from build123d import *

# Parameters (mm, degrees)
SKETCH1_W           = 25.4
SKETCH1_H           = 82.55
BOSS_EXTRUDE1_DEPTH = 3.175
SKETCH2_W           = 25.4
SKETCH2_H           = 3.175
SKETCH2_H_2         = 60.325
BOSS_EXTRUDE2_DEPTH = 3.175
SKETCH5_W           = 9.525
SKETCH5_H           = 19.05
CUT_EXTRUDE2_DEPTH  = 64.5
SKETCH6_R           = 3.175
CUT_EXTRUDE3_DEPTH  = 89.9


with BuildPart() as part:
    # Sketch1 → Boss-Extrude1 (new body)
    with BuildSketch(Plane.XY):
        Rectangle(SKETCH1_W, SKETCH1_H)
    extrude(amount=BOSS_EXTRUDE1_DEPTH)

    # Sketch2 → Boss-Extrude2 (add)
    with BuildSketch(Plane(origin=(0, 41.275, 0), x_dir=(1, 0, 0), z_dir=(0, 1, 0))):
        with Locations((0, -1.5875)):
            Rectangle(SKETCH2_W, SKETCH2_H)
        with Locations((0, 30.1625)):
            Rectangle(SKETCH2_W, SKETCH2_H_2)
    boss_extrude2 = extrude(amount=BOSS_EXTRUDE2_DEPTH)

    # Sketch5 → Cut-Extrude2 (cut, through all)
    with BuildSketch(Plane.XY.offset(3.175)):
        with Locations((0, 3.175)):
            Rectangle(SKETCH5_W, SKETCH5_H)
    extrude(amount=-CUT_EXTRUDE2_DEPTH, mode=Mode.SUBTRACT)

    # Mirror1: Boss-Extrude2 across plane
    add(boss_extrude2.mirror(Plane.ZX))

    # Sketch6 → Cut-Extrude3 (cut, through all)
    with BuildSketch(Plane(origin=(0, 44.45, 0), x_dir=(1, 0, 0), z_dir=(0, 1, 0))):
        with Locations((0, 49.2125)):
            Circle(SKETCH6_R)
    extrude(amount=-CUT_EXTRUDE3_DEPTH, mode=Mode.SUBTRACT)


solid = part.part
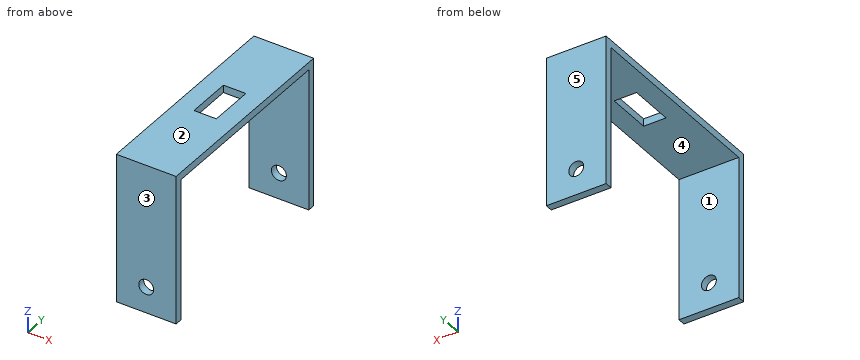
Read the model definition and answer for the solid it produces. Units are mm, in the model's axes. Face numbers are marked on the shaded views. A direction names the side the tool comes from. Round coordinates to 2 decimals unless told otherwise and drop trailing zeros. Write each loop counter-clockwise with the first axis right and the second up, starting at its lowest first coordinate (ties: lowest second). Pieces come first, ordered by that corner, then holes.
1. The part is cut by section D-D, the plane x = -7.75. Determine the outline of the cut face in (y, z) (3 decimals), then the cut area to 3 significant figures.
2. Determine the mould class of the marked faces 3, 4 and 5 for opening direction Y: pulls with the +Y half, pulls with the -Y half, needs draft (parallel to the pull), parting line crosses it, or undercut.
3. The part is cut by section A-A, the plane z = -31.5. Determine the outline of the cut face in (x, y) (3 decimals), then the cut area to 3 significant figures.
4. The part is cut by section B-B, the plane x = 0. State how many separate pieces and enclosed holes the cut face has, then the cut area to 3 significant figures.
5. The part is cut by section C-C, the plane y = -4. Determine the outline of the cut face in (x, z) (1 decimal), then the cut area to 3 significant figures.
6. Straight lines are drawn through the part: L1, parallel to Y at x = 3.25, z = -24 (3 decimals); L2, parallel to Z at x = 0, y = 42.9 (1 decimal); L3, parallel to Z at x = -8, y = -10 (3 decimals). For each, find the intervals that lie inside material, in ascending order.
7. Given pin 1 Ø3 at (x, y) = (-8, 7) entering from -Z; pin 2 Ø8 at (y, z) = (-8, -7) entering from -X, each flat-ended and moving along its own axis, determine where each tip first touches the part or whether it passes through.
8. Which of the six approach directions +Z, -Z, +X, -X, +Y, -Y give full straight-line access (tool end or side, diameter ignored) to the marked faces 1 and 2?
Values:
1. outline: (-44.45, -60.325) - (-41.275, -60.325) - (-41.275, 0) - (41.275, 0) - (41.275, -60.325) - (44.45, -60.325) - (44.45, 3.175) - (-44.45, 3.175) - close
1. area: 665 mm2
2. face 3: pulls with the -Y half
2. face 4: undercut
2. face 5: pulls with the +Y half
3. outline: (-12.7, -44.45) - (12.7, -44.45) - (12.7, -41.275) - (-12.7, -41.275) - close; (-12.7, 41.275) - (12.7, 41.275) - (12.7, 44.45) - (-12.7, 44.45) - close
3. area: 161 mm2
4. separate pieces: 4
4. enclosed holes: 0
4. area: 565 mm2
5. outline: (-12.7, 0) - (-4.8, 0) - (-4.8, 3.2) - (-12.7, 3.2) - close; (4.8, 0) - (12.7, 0) - (12.7, 3.2) - (4.8, 3.2) - close
5. area: 50.4 mm2
6. L1: y = -44.45 to -41.275, 41.275 to 44.45
6. L2: z = -60.3 to -52.4, -46 to 3.2
6. L3: z = 0 to 3.175
7. pin 1: stops at z = 0
7. pin 2: passes through
8. face 1: -Z, +X, -X
8. face 2: +Z, +X, -X, +Y, -Y
